```python
from build123d import *

# Parameters (mm, degrees)
SKETCH_2_W          = 115
SKETCH_2_H          = 40
EXTRUDE_1_DEPTH     = 25
SKETCH_3_W          = 100
SKETCH_3_H          = 40
CUT_EXTRUDE_1_DEPTH = 21
SKETCH_5_R          = 2
CUT_EXTRUDE_2_DEPTH = 138
FILLET_1_R          = 2
FILLET_2_R          = 2
SKETCH_6_R          = 4
CUT_EXTRUDE_3_DEPTH = 9
SKETCH_7_W          = 115
SKETCH_7_H          = 40
CUT_EXTRUDE_4_DEPTH = 3


with BuildPart() as part:
    # 草图2 → 凸台-拉伸1 (new body)
    with BuildSketch(Plane.XY):
        Rectangle(SKETCH_2_W, SKETCH_2_H)
    extrude(amount=EXTRUDE_1_DEPTH)

    # 草图3 → 切除-拉伸1 (cut)
    with BuildSketch(Plane.XY.offset(25)):
        Rectangle(SKETCH_3_W, SKETCH_3_H)
    extrude(amount=-CUT_EXTRUDE_1_DEPTH, mode=Mode.SUBTRACT)

    # 草图5 → 切除-拉伸2 (cut)
    with BuildSketch(Plane.ZY.offset(57.5)):
        with Locations(Location((10, 0, 0), (0, 0, 270))):
            Circle(SKETCH_5_R)
    extrude(amount=-CUT_EXTRUDE_2_DEPTH, mode=Mode.SUBTRACT)

    # 圆角1
    fillet_1_edges = [part.edges().sort_by_distance(p)[0] for p in [
        (0, 20, 0),
    ]]
    fillet(fillet_1_edges, radius=FILLET_1_R)

    # 圆角2
    fillet_2_edges = [part.edges().sort_by_distance(p)[0] for p in [
        (0, -20, 0),
    ]]
    fillet(fillet_2_edges, radius=FILLET_2_R)

    # 草图6 → 切除-拉伸3 (cut)
    with BuildSketch(Plane.XY.offset(4)):
        with Locations((-25, 0)):
            Circle(SKETCH_6_R)
        with Locations(Location((25, 0, 0), (0, 0, 180))):
            Circle(SKETCH_6_R)
    extrude(amount=-CUT_EXTRUDE_3_DEPTH, mode=Mode.SUBTRACT)

    # 草图7 → 切除-拉伸4 (cut)
    with BuildSketch(Plane.XY.offset(25)):
        Rectangle(SKETCH_7_W, SKETCH_7_H)
    extrude(amount=-CUT_EXTRUDE_4_DEPTH, mode=Mode.SUBTRACT)


solid = part.part
```
Here's how the part is built. I have some questions about the finished solid (model axes, mm). A direction names the side the tool comes from. Give positions to 0.01 mm unless a question says otherwise; leave off trailing zeros. Order: outer loops, then holes, each group sorted by start corner. A loop starts at its lowest first (then second) coordinate and runs counter-clockwise, first axis right, second up. Notation, with made-up numbers: (-37, 38.5) - (-26, 38.5) arc R11 cw to (-26, 42.5) - close; hole circle Ø2 at (40.5, 82). An arc over 180 degrees is marked (long way). Answer as a JSON object with one key per item and string values. Group by question number.
Item 1: Which directions (+Z, -Z, +X, -X, +Y, -Y) give clear straight access to the entire face, cutting with the end or side of a thin tool? Please do faces 1 (the flat face through (-57.5, 0, 13)), 2 (the flat face through (-50, 0, 13)).
Item 2: For P1, Ø1, axis at x = 17, y = 13, coming from the +Z side; P2, Ø6.5, axis at x = -25, y = 0, coming from the -Z side, each with a flat end and sliding along its axis, tell me the tip position at first contact or that it passes through.
Item 3: If we section it at C-C on x = -25: Please give me the cut outline in (y, z), and give its area (3 significant figures).
Item 4: Please list where these lines run through material, in increasing order: probe 1 along X at (y, z) = (14.5, 7.5); probe 2 along Z at (x, y) = (-55.5, 0); probe 3 along Y at (x, z) = (-25, 2.5).
Item 5: If we section it at A-A on y = 0: Please give me the cut outline in (x, z).
Item 6: If we section it at B-B on z = 6.5: Please give me the cut outline in (x, y).
Item 7: If we mould it in two halves opening along Z, with no side actions, what happens to faces 3 (the flat face through (-54, 0, 22)), 4 (the cylindrical face through (54, 0, 12)), 5 (the flat face through (-0.3, 20, 3.8)), 6 (the cylindrical face through (-54, 0, 12))? For each: pulls with the +Z half, pulls with the -Z half, needs draft (parallel to the pull), parting line crosses it, or undercut.
Item 8: If we section it at D-D on y = -8.5: Please give me the cut outline in (x, z).
Result set:
{
 "1": {"face 1": "+Z, -Z, -X, +Y, -Y", "face 2": "+Z, +Y, -Y"},
 "2": {"P1": "z = 4", "P2": "through"},
 "3": {"outline": "(-20, 2) arc R2 ccw to (-18, 0) - (-4, 0) - (-4, 4) - (-20, 4) - close; (4, 0) - (18, 0) arc R2 ccw to (20, 2) - (20, 4) - (4, 4) - close", "area": "126 mm²"},
 "4": {"probe 1": "-57.5 to -50, 50 to 57.5", "probe 2": "0 to 8, 12 to 22", "probe 3": "-20 to -4, 4 to 20"},
 "5": {"outline": "(-57.5, 0) - (-29, 0) - (-29, 4) - (-50, 4) - (-50, 8) - (-57.5, 8) - close; (-57.5, 12) - (-50, 12) - (-50, 22) - (-57.5, 22) - close; (-21, 0) - (21, 0) - (21, 4) - (-21, 4) - close; (29, 0) - (57.5, 0) - (57.5, 8) - (50, 8) - (50, 4) - (29, 4) - close; (50, 12) - (57.5, 12) - (57.5, 22) - (50, 22) - close"},
 "6": {"outline": "(-57.5, -20) - (-50, -20) - (-50, 20) - (-57.5, 20) - close; (50, -20) - (57.5, -20) - (57.5, 20) - (50, 20) - close"},
 "7": {"face 3": "pulls with the +Z half", "face 4": "undercut", "face 5": "needs draft", "face 6": "undercut"},
 "8": {"outline": "(-57.5, 0) - (57.5, 0) - (57.5, 22) - (50, 22) - (50, 4) - (-50, 4) - (-50, 22) - (-57.5, 22) - close"}
}
